from build123d import *

# Parameters (mm, degrees)
BOSS_EXTRUDE1_DEPTH      = 12
SKETCH2_R                = 2
CUT_EXTRUDE1_DEPTH       = 244.893675605
SKETCH3_W                = 47.3
SKETCH3_H                = 27.3
SKETCH3_W_2              = 27.3
SKETCH3_H_2              = 47.3
CUT_EXTRUDE2_DEPTH       = 7
CUT_EXTRUDE8_DEPTH       = 244.893675605
CUT_EXTRUDE8_DEPTH_BACK  = 244.893675605
SKETCH5_R                = 1.95
SKETCH5_R_2              = 2
CUT_EXTRUDE10_DEPTH      = 244.893675605
CUT_EXTRUDE10_DEPTH_BACK = 244.893675605
SKETCH9_W                = 10
SKETCH9_H                = 9.75
SKETCH9_W_2              = 9.75
SKETCH9_H_2              = 10
CUT_EXTRUDE11_DEPTH      = 244.522201247
FILLET1_R                = 1


# Read off the part's stored shape, not the designer's step: Boss-Extrude1
with BuildPart() as part:
    # Boss-Extrude1 outline → Boss-Extrude1 (new body)
    with BuildSketch(Plane(origin=(0, 0, 0), x_dir=(1, 0, 0), z_dir=(0, 1, 0))):
        Polygon((0, 0), (0, -17.25), (155, -172.25), (172.25, -172.25), (172.25, -152.25), (20, 0), align=None)
    extrude(amount=BOSS_EXTRUDE1_DEPTH)

    # Sketch2 → Cut-Extrude1 (cut, through all)
    with BuildSketch(Plane(origin=(0, 12, 0), x_dir=(1, 0, 0), z_dir=(0, 1, 0))):
        with Locations(Location((10, -16.25, 0), (0, 0, 270))):
            Circle(SKETCH2_R)
        with Locations(Location((156, -162.25, 0), (0, 0, 270))):
            Circle(SKETCH2_R)
    extrude(amount=-CUT_EXTRUDE1_DEPTH, mode=Mode.SUBTRACT)

    # Sketch3 → Cut-Extrude2 (cut)
    with BuildSketch(Plane(origin=(0, 12, 0), x_dir=(1, 0, 0), z_dir=(0, 1, 0))):
        with Locations((23.65, -13.65)):
            Rectangle(SKETCH3_W, SKETCH3_H)
        with Locations((158.6, -148.6)):
            Rectangle(SKETCH3_W_2, SKETCH3_H_2)
    extrude(amount=-CUT_EXTRUDE2_DEPTH, mode=Mode.SUBTRACT)

    # Sketch5 → Cut-Extrude8 (cut, two sides: drawn at the far end of the back side and taken through both)
    with BuildSketch(Plane(origin=(0, 0, 0), x_dir=(1, 0, 0), z_dir=(0, 1, 0)).offset(-CUT_EXTRUDE8_DEPTH_BACK)):
        with Locations(Location((128.411688245, -128.691125497, 0), (0, 0, 270))):
            Circle(SKETCH5_R)
        with Locations(Location((107.19848481, -107.477922061, 0), (0, 0, 270))):
            Circle(SKETCH5_R_2)
        with Locations(Location((43.558874503, -43.838311755, 0), (0, 0, 90))):
            Circle(SKETCH5_R)
        with Locations(Location((64.772077939, -65.05151519, 0), (0, 0, 90))):
            Circle(SKETCH5_R_2)
    extrude(amount=CUT_EXTRUDE8_DEPTH + CUT_EXTRUDE8_DEPTH_BACK, mode=Mode.SUBTRACT)

    # Sketch8 → Cut-Extrude10 (cut, two sides: drawn at the far end of the back side and taken through both)
    with BuildSketch(Plane.XZ.offset(-CUT_EXTRUDE10_DEPTH_BACK)):
        Polygon((0, 497.196572238), (0, 0), (0, -10), (182, -10), (182, 172.25), (172, 172.25), (172, 152.353553391), (19.896446609, 0.25), (0, 0.25), (-497.196572238, 0.25), (205.768720009, -703.068934535), (702.965292247, -206.122362298), align=None)
    extrude(amount=CUT_EXTRUDE10_DEPTH + CUT_EXTRUDE10_DEPTH_BACK, mode=Mode.SUBTRACT)

    # Sketch9 → Cut-Extrude11 (cut, through all)
    with BuildSketch(Plane(origin=(0, 5, 0), x_dir=(1, 0, 0), z_dir=(0, 1, 0))):
        with Locations((10, -5.125)):
            Rectangle(SKETCH9_W, SKETCH9_H)
        with Locations((167.125, -162.25)):
            Rectangle(SKETCH9_W_2, SKETCH9_H_2)
    extrude(amount=-CUT_EXTRUDE11_DEPTH, mode=Mode.SUBTRACT)

    # Fillet1
    fillet1_edges = [part.edges().sort_by_distance(p)[0] for p in [
        (5, 2.5, 10),
        (15, 2.5, 10),
        (162.25, 2.5, 167.25),
        (162.25, 2.5, 157.25),
    ]]
    fillet(fillet1_edges, radius=FILLET1_R)


solid = part.part
Read the model definition and answer for the solid it produces. Units are mm, in the model's axes. A direction names the side the tool comes from. Coordinates: 2 decimals unless noted, no trailing zeros. Order: outer loops, then holes, each group sorted by start corner. A loop starts at its lowest first (then second) coordinate and runs counter-clockwise, first axis right, second up. Notation, with made-up numbers: M -27.75,27 L 9.25,27 A27 ccw 9.25,53 Z; hole C 71,37 d2. An arc over 180 degrees is marked long. Put each result on its own line as item: value. Start each with the question number.
Item 1: Given pin 1 Ø3 at (y, z) = (2, 84.5) entering from +X; pin 2 Ø1.5 at (y, z) = (3, 164) entering from +X; pin 3 Ø6 at (y, z) = (7.5, 143) entering from +X, each flat-ended and moving along its own axis, determine where each tip first touches the part or whether it passes through.
Item 2: Section A-A, the plane z = 134 is taken. Determine the outline of the cut face in (x, y), plus the area to 3 significant figures.
Item 3: Consider probe 1 along Z at (x, y) = (156, 2.25); probe 2 along Z at (x, y) = (107.5, 10.5); probe 3 along X at (y, z) = (1.3, 162.25). Determine where each line is inside the solid, lowest interval first. Write a range as [from, to].
Item 4: The mould has two halves that part along Z. Classify faces 4 (the face through (87, 12, 84)), 5 (the face through (11.983, 2.535, 15.99)), 6 (the face through (163, 2, 172.25)): +Z half, -Z half, draft (parallel to the pull), parting line (faces both ways), or undercut.
Item 5: For faces 1 (the face through (168, 3, 167.25)), 2 (the face through (28, 9, 27.3)), 3 (the face through (5, 3, 5)), determine the directions among +Z, -Z, +X, -X, +Y, -Y from which every point of the face is accessible in a straight line to the end or side of a thin tool.
Item 6: Section B-B, the plane z = 112 is taken. Determine the outline of the cut face in (x, y).
Computed:
1. pin 1: stops at x = 105.65
1. pin 2: stops at x = 162.25
1. pin 3: stops at x = 164.3
2. outline: M 116.75,0 L 153.65,0 L 153.65,5 L 144.95,5 L 144.95,12 L 116.75,12 Z
2. area: 382 mm2
3. probe 1: z = [136.35, 160.25], [164.25, 172.25]
3. probe 2: z = [87.85, 105.5], [109.46, 124.75]
3. probe 3: x = [145, 154], [158, 162.25]
4. face 4: draft
4. face 5: undercut
4. face 6: +Z half
5. face 1: +X, +Y, -Y
5. face 2: -Z, +X, -X, +Y
5. face 3: -Z, +Y, -Y
6. outline: M 94.75,0 L 131.65,0 L 131.65,12 L 94.75,12 Z
